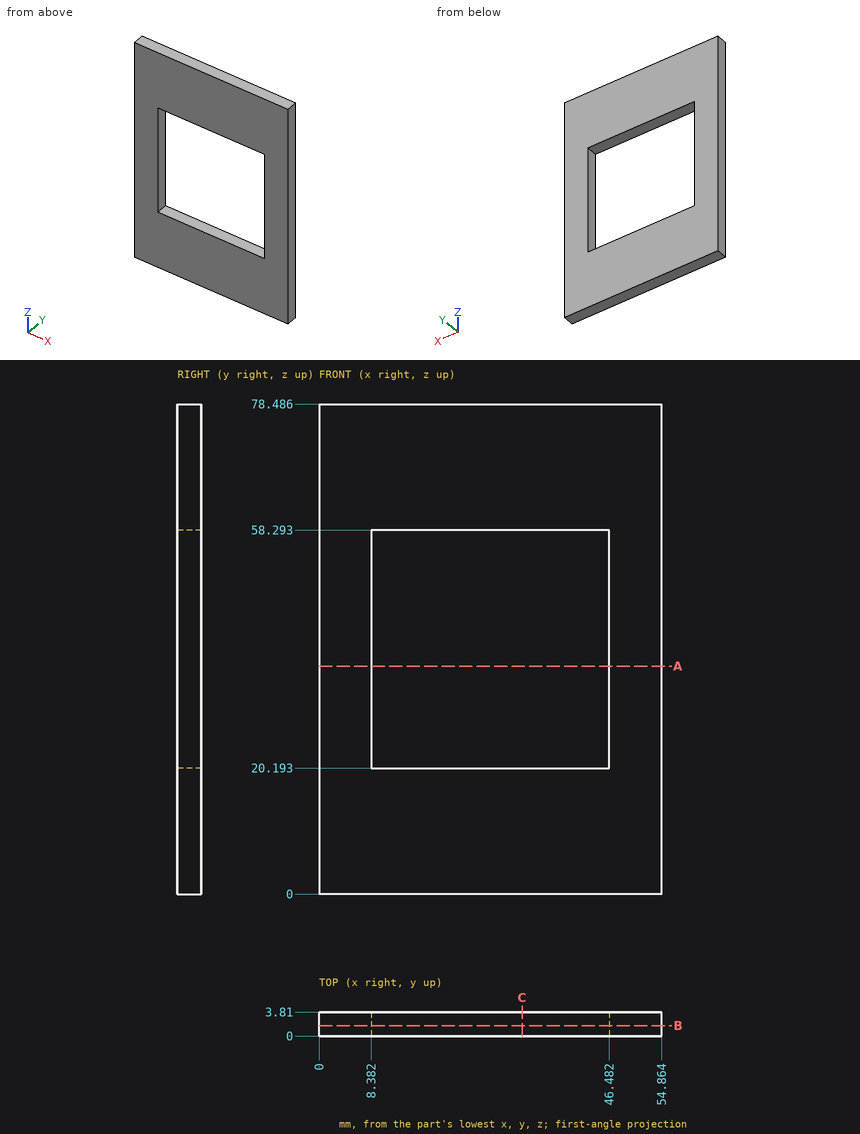
Can you work these out from the drawing? Everything is in mm from the part's minimum corner. Give positions to 0.01 mm unless a question says otherwise; leave off trailing zeros. Loops run counter-clockwise (first coordinate to the right, second up) from the corner with the lowest first, then second, coordinate; pieces in that order, holes last. Notation, with made-up numbers: M 31,76.5 L 45,76.5 A17 ccw 45,108.5 Z; hole C 43.5,37.5 d6. An arc over 180 degrees is marked long. Put each result on its own line as item: value. Start each with the question number.
(1) I want a section at B-B on y = 1.65. Please give me the cut outline in (x, z), then the cut area to 3 significant figures.
(2) I need wall thicknesses on line 1 along X through (y, z) = (2.45, 47); line 2 along Z through (x, y) = (12, 3.3). Which ranges of each line are inside material? Lowest first, please. Write a range as [from, to].
(3) I want a section at A-A on z = 36.5. Please give me the cut outline in (x, y).
(4) I want a section at C-C on x = 32.5. Please give me the cut outline in (y, z).
Answer block:
1. outline: M 0,0 L 54.86,0 L 54.86,78.49 L 0,78.49 Z; hole M 8.38,20.19 L 46.48,20.19 L 46.48,58.29 L 8.38,58.29 Z
1. area: 2,850 mm^2
2. line 1: [0, 8.38], [46.48, 54.86]
2. line 2: [0, 20.19], [58.29, 78.49]
3. outline: M 0,0 L 8.38,0 L 8.38,3.81 L 0,3.81 Z; M 46.48,0 L 54.86,0 L 54.86,3.81 L 46.48,3.81 Z
4. outline: M 0,0 L 3.81,0 L 3.81,20.19 L 0,20.19 Z; M 0,58.29 L 3.81,58.29 L 3.81,78.49 L 0,78.49 Z
